The model under review builds one solid part; all positions refer to its coordinate system, in mm. Face numbers are marked on the shaded views. A direction names the side the tool comes from. Give positions to 0.01 mm unless a question says otherwise; leave off trailing zeros. Order: outer loops, then holes, each group sorted by start corner. A loop starts at its lowest first (then second) coordinate and runs counter-clockwise, first axis right, second up. Notation, with made-up numbers: (-40, 52.5) - (-1, 52.5) arc R15 ccw to (-1, 81.5) - close; hole circle Ø1 at (1.25, 79.5). An arc over 180 degrees is marked (long way). Use CSV: the item, a comma, the result in double quotes.
```python
from build123d import *

# Parameters (mm, degrees)
CROQUIS1_W              = 40
CROQUIS1_H              = 40
CROQUIS1_W_2            = 39
CROQUIS1_H_2            = 39
SALIENTE_EXTRUIR2_DEPTH = 300
CORTAR_EXTRUIR1_DEPTH   = 300
CORTAR_EXTRUIR2_DEPTH   = 300
CROQUIS4_R              = 1.5
CORTAR_EXTRUIR3_DEPTH   = 550


with BuildPart() as part:
    # Croquis1 → Saliente-Extruir2 (new body)
    with BuildSketch(Plane.XY):
        Rectangle(CROQUIS1_W, CROQUIS1_H)
        Rectangle(CROQUIS1_W_2, CROQUIS1_H_2, mode=Mode.SUBTRACT)
    extrude(amount=SALIENTE_EXTRUIR2_DEPTH)

    # Croquis2 → Cortar-Extruir1 (cut)
    with BuildSketch(Plane(origin=(0, 20, 0), x_dir=(1, 0, 0), z_dir=(0, 1, 0))):
        Polygon((-19.5, -300), (20, -260.5), (20, -300), align=None)
    extrude(amount=-CORTAR_EXTRUIR1_DEPTH, mode=Mode.SUBTRACT)

    # Croquis3 → Cortar-Extruir2 (cut)
    with BuildSketch(Plane.XZ.offset(20)):
        Polygon((-20, 0), (20, 40), (20, 0), align=None)
    extrude(amount=-CORTAR_EXTRUIR2_DEPTH, mode=Mode.SUBTRACT)

    # Croquis4 → Cortar-Extruir3 (cut)
    with BuildSketch(Plane.XZ.offset(20)):
        with Locations(Location((0, 45, 0), (0, 0, 270))):
            Circle(CROQUIS4_R)
        with Locations(Location((0, 90, 0), (0, 0, 270))):
            Circle(CROQUIS4_R)
        with Locations(Location((0, 135, 0), (0, 0, 270))):
            Circle(CROQUIS4_R)
        with Locations(Location((0, 180, 0), (0, 0, 270))):
            Circle(CROQUIS4_R)
        with Locations(Location((0, 225, 0), (0, 0, 270))):
            Circle(CROQUIS4_R)
        with Locations(Location((0, 270, 0), (0, 0, 270))):
            Circle(CROQUIS4_R)
    extrude(amount=-CORTAR_EXTRUIR3_DEPTH, mode=Mode.SUBTRACT)


solid = part.part
```
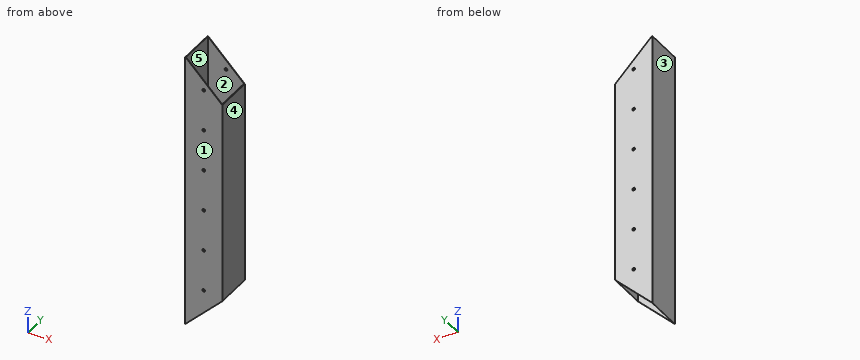
Item 1: Mouldability with a two-part tool opening along X and no side actions: class the marked faces 3, 4 and 5 as pulls with the +X half, pulls with the -X half, needs draft (parallel to the pull), parting line crosses it, or undercut.
Results list:
face 3,"pulls with the -X half"
face 4,"pulls with the +X half"
face 5,"undercut"
Item 2: Tool access review of the marked faces 1 and 2: name each direction out of +Z, -Z, +X, -X, +Y, -Y from which nothing blocks a thin tool from reaching the whole face with its end or side.
Results list:
face 1,"+Z, -Z, +X, -X, -Y"
face 2,"+Z, -Z"
Item 3: Wall thickness on L1, parallel to X at y = 16, z = 50.5; L2, parallel to X at y = -19.7, z = 180: over which ranges is each line inside the solid? List them lowest first.
Results list:
L1,"x = -20 to -19.5, 19.5 to 20"
L2,"x = -20 to -1.5, 1.5 to 20"
Item 4: Clearance check with flat-ended pins moving along their axes: pin 1 (12 mm diameter, centred on x = 12.5, y = 11, fed in from +Z); pin 2 (4 mm diameter, centred on x = 0, z = 90, fed in from +Y). State where each tip first meets the part, or that it passes through.
Results list:
pin 1,"passes through"
pin 2,"stops at y = 20"
Item 5: Take a section at C-C, the plane z = 129. Give the boundary of the cut face in (x, y).
Results list:
outline,"(-20, -20) - (20, -20) - (20, 20) - (-20, 20) - close; hole (-19.5, -19.5) - (19.5, -19.5) - (19.5, 19.5) - (-19.5, 19.5) - close"
Item 6: Take a section at A-A, the plane x = 17. Give the boundary of the cut face in (y, z).
Results list:
outline,"(-20, 37) - (-19.5, 37) - (-19.5, 263.5) - (-20, 263.5) - close; (19.5, 37) - (20, 37) - (20, 263.5) - (19.5, 263.5) - close"
Item 7: Take a section at B-B, the plane y = 15.5. Give the boundary of the cut face in (x, z), and give its area (3 significant figures).
Results list:
outline,"(-20, 0) - (-19.5, 0.5) - (-19.5, 300) - (-20, 300) - close; (19.5, 39.5) - (20, 40) - (20, 260.5) - (19.5, 261) - close"
area,"260 mm2"
